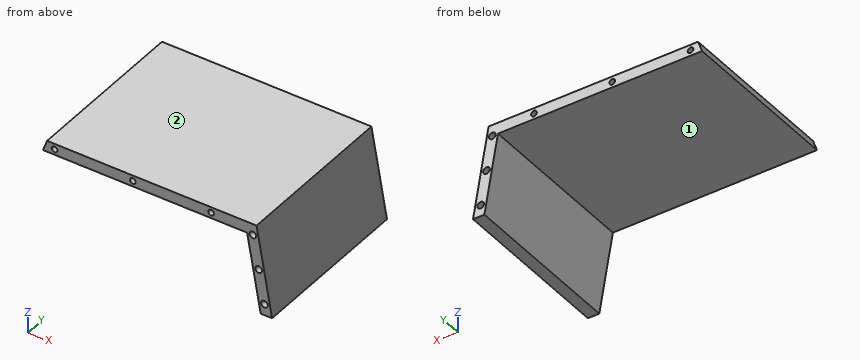
```python
from build123d import *

# Parameters (mm, degrees)
BOSS_EXTRUDE1_DEPTH = 37.5
SKETCH2_R           = 1.271589992
SKETCH2_R_2         = 1.5
CUT_EXTRUDE1_DEPTH  = 15


with BuildPart() as part:
    # Sketch1 → Boss-Extrude1 (new body)
    with BuildSketch(Plane(origin=(0, 0, 0), x_dir=(-1, 0, 0), z_dir=(0, 1, 0))):
        Polygon((28.132122167, -13), (-65.526137841, -13), (-72.491053579, -52.5), (-67.41392052, -52.5), (-61.330639685, -18), (29.951973339, -18), align=None)
    extrude(amount=BOSS_EXTRUDE1_DEPTH)

    # Sketch2 → Cut-Extrude1 (cut)
    with BuildSketch(Plane(origin=(0, 37.5, 0), x_dir=(-1, 0, 0), z_dir=(0, 1, 0))):
        with Locations(Location((-45.214663337, -15.5, 0), (0, 0, 90))):
            Circle(SKETCH2_R)
        with Locations(Location((-10.214663337, -15.5, 0), (0, 0, 90))):
            Circle(SKETCH2_R)
        with Locations(Location((24.785336663, -15.5, 0), (0, 0, 90))):
            Circle(SKETCH2_R)
        with Locations(Location((-69.070852146, -47.5, 0), (0, 0, 90))):
            Circle(SKETCH2_R_2)
        with Locations(Location((-66.466129481, -32.727883705, 0), (0, 0, 90))):
            Circle(SKETCH2_R_2)
        with Locations(Location((-63.861406816, -17.95576741, 0), (0, 0, 90))):
            Circle(SKETCH2_R_2)
    extrude(amount=-CUT_EXTRUDE1_DEPTH, mode=Mode.SUBTRACT)

    # Mirror1: part across plane


with BuildPart() as part_1:
    add(part.part)
    add(part.part.mirror(Plane(origin=(0, 0, 0), x_dir=(0, 0, 1), z_dir=(0, -1, 0))))


solid = part_1.part
```
Here's how the part is built. I have some questions about the finished solid (model axes, mm). Face numbers are marked on the shaded views. A direction names the side the tool comes from. Give positions to 0.01 mm unless a question says otherwise; leave off trailing zeros. Order: outer loops, then holes, each group sorted by start corner. A loop starts at its lowest first (then second) coordinate and runs counter-clockwise, first axis right, second up. Notation, with made-up numbers: M 71,46.25 L 113,46.25 A18 cw 113,63.25 Z; hole C 19.5,45 d10. An arc over 180 degrees is marked long. Use a Markdown table: item, result. Add a question column.
1. Suppose I cut it at D-D (z = -47.5). List the corners of the cut face in (x, y) for me, and give its area (3 significant figures).
2. Suppose I cut it at B-B (y = -5). List the corners of the cut face in (x, z) for me.
3. On a 3-axis mill with a long thin cutter (end or side, diameter ignored), from which of +Z, -Z, +X, -X, +Y, -Y can I reach the whole of each face in a straight line? I mean the marked faces 1 and 2. Say none if no direction works.
4. I need wall thicknesses on probe 1 along X at (y, z) = (33.5, -15.5); probe 2 along Z at (x, y) = (8, -30); probe 3 along X at (y, z) = (34, -15). Which ranges of each line are inside material? Lowest first, please. Write a range as from..to.
5. Suppose I cut it at A-A (y = -26.5). List the corners of the cut face in (x, z) for me.
6. For pin 1 Ø1.5 at (y, z) = (-14.5, -32.5) entering from -X; pin 2 Ø1.8 at (x, z) = (69.07, -47.5) entering from -Y; pin 3 Ø1.5 at (y, z) = (-14.5, -23.5) entering from +X, each with a flat end and sliding along its axis, tell me the tip position at first contact or that it passes through.
7. Suppose I cut it at C-C (x = 28). List the corners of the cut face in (y, z) for me, and give its area (3 significant figures).
Results list:
| question | item | result |
|---|---|---|
| 1 | outline | M 66.53,-37.5 L 67.57,-37.5 L 67.57,-22.5 L 70.57,-22.5 L 70.57,-37.5 L 71.61,-37.5 L 71.61,37.5 L 70.57,37.5 L 70.57,22.5 L 67.57,22.5 L 67.57,37.5 L 66.53,37.5 Z |
| 1 | area | 291 mm² |
| 2 | outline | M -29.95,-18 L 61.33,-18 L 67.41,-52.5 L 72.49,-52.5 L 65.53,-13 L -28.13,-13 Z |
| 3 | face 1 | -Z, -X, +Y, -Y |
| 3 | face 2 | +Z, +X, -X, +Y, -Y |
| 4 | probe 1 | x = -29.04..-26.06, -23.51..8.94, 11.49..43.94, 46.49..65.97 |
| 4 | probe 2 | z = -18..-13 |
| 4 | probe 3 | x = -28.86..-25.95, -23.62..9.05, 11.38..44.05, 46.38..65.88 |
| 5 | outline | M -29.95,-18 L 61.33,-18 L 67.41,-52.5 L 72.49,-52.5 L 65.53,-13 L -28.13,-13 Z; hole C -24.79,-15.5 d2.54; hole C 10.21,-15.5 d2.54; hole C 45.21,-15.5 d2.54; hole C 63.86,-17.96 d3; hole C 66.47,-32.73 d3; hole C 69.07,-47.5 d3 |
| 6 | pin 1 | stops at x = 63.76 |
| 6 | pin 2 | stops at y = -22.5 |
| 6 | pin 3 | stops at x = 67.51 |
| 7 | outline | M -37.5,-18 L 37.5,-18 L 37.5,-13 L -37.5,-13 Z |
| 7 | area | 375 mm² |
